Read the model definition and answer for the solid it produces. Units are mm, in the model's axes. A direction names the side the tool comes from. Coordinates: 2 decimals unless noted, no trailing zeros. Order: outer loops, then holes, each group sorted by start corner. A loop starts at its lowest first (then second) coordinate and runs counter-clockwise, first axis right, second up.
Autodesk Inventor part; units mm, degrees
ref_plane "작업 평면1" through (-21.25, -9.325, 0) normal (0, -1, 0) x (1, 0, 0)
ref_plane "YZ Plane" through (0, 0, 0) normal (1, 0, 0) x (0, 1, 0)
ref_plane "XZ Plane" through (0, 0, 0) normal (0, 1, 0) x (-1, 0, 0)
sketch "스케치1" plane through (0, 0, 0) normal (0, 0, 1) x (1, 0, 0)
  line L0 (-21.25, 18.125) -> (21.25, 18.125)
  line L1 (21.25, 18.125) -> (21.25, -18.125)
  line L2 (21.25, -18.125) -> (-21.25, -18.125)
  line L3 (-21.25, -18.125) -> (-21.25, 18.125)
  line L4 (-21.25, 18.125) -> (21.25, -18.125) construction
  line L5 (21.25, 18.125) -> (-21.25, -18.125) construction
  point P0 (0, 0)
  dimension "d0" = 42.5
  dimension "d1" = 36.25
extrude "돌출1" add sketch "스케치1" along normal blind 3
fillet "모깎기1" radius 5 2 edges at (21.25, 18.125, 1.5) (-21.25, 18.125, 1.5)
ref_plane "작업 평면1" through (-21.25, -9.325, 0) normal (0, -1, 0) x (1, 0, 0)
sketch "스케치2" plane through (-21.25, -9.325, 0) normal (0, -1, 0) x (1, 0, 0)
  line L0 (21.25, 0) -> (21.25, -4)
  circle A0 centre (21.25, -4) radius 2
  circle A1 centre (21.25, -4) radius 4
  line L1 (21.25, 0) -> (26.25, 0)
  line L2 (0, 0) -> (42.5, 0) construction
  line L3 (26.25, 0) -> (25.1524, -4.878)
  line L4 (21.25, 0) -> (16.25, 0)
  line L5 (16.25, 0) -> (17.4292, -5.184)
  dimension "d6" = 4
  dimension "d7" = 4
  dimension "d8" = 8
  dimension "d9" = 10
extrude "돌출2" add sketch "스케치2" along normal blind 2 contours L1 L3 A1 | A1 L5 | A1 L5 L4 picked at (20.9261, -0.7066)
pattern_linear "직사각형 패턴1" count 2 spacing 22.5 along (0, 1, 0) of "돌출2"
sketch "스케치3" plane through (0, 0, 0) normal (0, 0, -1) x (-1, 0, 0)
  circle A0 centre (16.825, -2.325) radius 4.425
  line L0 (21.25, -18.125) -> (-21.25, -18.125)
  line L1 (0, 0) -> (0, 4.3779)
  circle A1 centre (-16.825, -2.325) radius 4.425
  line L2 (21.25, 13.125) -> (21.25, -18.125)
  line L3 (-19.075, -0.075) -> (-14.575, -0.075)
  line L4 (-14.575, -0.075) -> (-14.575, -4.575)
  line L5 (-14.575, -4.575) -> (-19.075, -4.575)
  line L6 (-19.075, -4.575) -> (-19.075, -0.075)
  line L7 (-19.075, -0.075) -> (-14.575, -4.575) construction
  line L8 (-14.575, -0.075) -> (-19.075, -4.575) construction
  line L9 (14.575, -4.575) -> (19.075, -4.575)
  line L10 (19.075, -4.575) -> (19.075, -0.075)
  line L11 (19.075, -0.075) -> (14.575, -0.075)
  line L12 (14.575, -0.075) -> (14.575, -4.575)
  line L13 (14.575, -4.575) -> (19.075, -0.075) construction
  line L14 (19.075, -4.575) -> (14.575, -0.075) construction
  dimension "d16" = 15.8
  dimension "d17" = 33.65
  dimension "d18" = 4.5
  dimension "d19" = 4.5
  dimension "d20" = 4.5
  dimension "d21" = 4.5
extrude "돌출3" add sketch "스케치3" along normal blind 2
sketch "스케치4" plane through (0, 0, 3) normal (0, 0, 1) x (1, 0, 0)
  line L0 (-21.25, -18.125) -> (21.25, -18.125)
  line L1 (21.25, -18.125) -> (21.25, 13.125)
  line L2 (-21.25, 13.125) -> (-21.25, -18.125)
  line L3 (-21.25, -17.625) -> (21.25, -17.625)
  point P0 (0, 0)
  dimension "d24" = 0.5
extrude "돌출4" cut sketch "스케치4" against normal blind 3
sketch "스케치5" plane through (0, 0, 3) normal (0, 0, 1) x (1, 0, 0)
  line L0 (-17, 7) -> (-15, 7)
  line L1 (-15, 7) -> (-15, -13)
  line L2 (-15, -13) -> (-17, -13)
  line L3 (-17, -13) -> (-17, 7)
  line L4 (-17, 7) -> (-15, -13) construction
  line L5 (-15, 7) -> (-17, -13) construction
  point P0 (0, 0)
  point P1 (-16, -3)
  dimension "d27" = 2
  dimension "d28" = 20
  dimension "d32" = 3
  dimension "d37" = 16
extrude "돌출5" cut sketch "스케치5" against normal blind 0.5
chamfer "모따기1" distance 0.5 angle 45 4 edges at (-17, -3, 3) (-16, 7, 3) (-15, -3, 3) (-16, -13, 3)
sketch "스케치6" plane through (0, 0, 0) normal (0, 0, -1) x (-1, 0, 0)
  line L0 (14.575, -4.575) -> (19.075, -4.575)
  line L1 (19.075, -4.575) -> (19.075, -0.075)
  line L2 (19.075, -0.075) -> (14.575, -0.075)
  line L3 (14.575, -0.075) -> (14.575, -4.575)
  line L4 (-19.075, -0.075) -> (-19.075, -4.575)
  line L5 (-19.075, -4.575) -> (-14.575, -4.575)
  line L6 (-14.575, -4.575) -> (-14.575, -0.075)
  line L7 (-14.575, -0.075) -> (-19.075, -0.075)
  point P0 (0, 0)
extrude "돌출6" add sketch "스케치6" along normal blind 0.3
sketch "스케치7" plane through (-5, 11.175, 0) normal (0, -1, 0) x (1, 0, 0)
  arc A0 (1.1792, -5.184) -> (8.9024, -4.878) centre (5, -4) ccw
  line L0 (8.9024, -4.878) -> (1.1096, -4.878)
  line L1 (1.1096, -4.878) -> (1.1096, -8)
  line L2 (1.1096, -8) -> (8.9024, -8)
  line L3 (8.9024, -8) -> (8.9024, -4.878)
  line L4 (0, 0) -> (1.1792, -5.184)
  point P0 (5, 0)
  point P1 (5, -8)
extrude "돌출7" add sketch "스케치7" against normal blind 2 contours A0 L2 L1 L4 | A0 L3 L2
pattern_linear "직사각형 패턴2" count 2 spacing 22.5 along (0, -1, 0) of "돌출7"
chamfer "모따기2" distance 1 angle 45 4 edges at (3.9024, 12.175, -8) (-3.8904, 12.175, -8) (3.9024, -10.325, -8) (-3.8904, -10.325, -8)
properties part number "버튼 스위치 상단"
Q1. The part is cut by section D-D, the plane x = 15.5. Determine the outline of the cut face in (y, z) (3 decimals), then the cut area to 3 significant figures.
Q2. Determine the mould class of faces 5 (the flat face through (17, -2, -0.3)), 6 (the flat face through (-17, -5, -2)), 7 (the flat face through (-17, -0.075, -1)), 8 (the flat face through (3.4, 12.2, -7.5)) for opening direction X: +X half, -X half, draft (parallel to the pull), parting line (faces both ways), or undercut.
Q3. The part is cut by section A-A, the plane x = 0. Determine the outline of the cut face in (y, z) (3 decimals), then the cut area to 3 significant figures.
Q4. Each of these flat-tipped pins is pushed along its axis until it touches: P1, Ø1, axis at y = 11.5, z = -5.5, coming from the -X side; P2, Ø6.5, axis at x = 1, z = -4, coming from the -Y side (3 decimals); P3, Ø7, axis at x = 15, y = -2.5, coming from the -Z side; P4, Ø1.9, axis at y = -3, z = -1, coming from the +X side. Where does it stop, or does it pass through?
Q5. The part is cut by section B-B, the plane z = -3.5. Determine the outline of the cut face in (x, y) (1 decimal).
Q6. Which of the six approach directions +Z, -Z, +X, -X, +Y, -Y give full straight-line access (tool end or side, diameter ignored) to faces 1 (the flat face through (1, 13.175, -2)), 2 (the flat face through (1, -9.325, -2)), 3 (the flat face through (3.902, -10, -6)), 4 (the flat face through (-14.575, -2, -1))?
Q7. Straight lines are drawn through the part: L1, parallel to Z at x = 0, y = -10.5; L2, parallel to Y at x = -3, z = -5.75 (3 decimals); L3, parallel to Z at x = -17.5, y = -5.5. For each, find the intervals that lie inside material, in ascending order.
Computed values:
1. outline: (-17.625, 0) - (-6.547, 0) - (-6.547, -2) - (-4.575, -2) - (-4.575, -0.3) - (-0.075, -0.3) - (-0.075, -2) - (1.897, -2) - (1.897, 0) - (18.125, 0) - (18.125, 3) - (-17.625, 3) - close
1. area: 116 mm2
2. face 5: undercut
2. face 6: draft
2. face 7: undercut
2. face 8: +X half
3. outline: (-17.625, 0) - (-11.325, 0) - (-11.325, -2) - (-9.325, -2) - (-9.325, 0) - (11.175, 0) - (11.175, -2) - (13.175, -2) - (13.175, 0) - (18.125, 0) - (18.125, 3) - (-17.625, 3) - close; (-11.325, -8) - (-9.325, -8) - (-9.325, -6) - (-11.325, -6) - close; (11.175, -8) - (13.175, -8) - (13.175, -6) - (11.175, -6) - close
3. area: 123 mm2
4. P1: stops at x = -3.89
4. P2: stops at y = -11.325
4. P3: stops at z = -2
4. P4: stops at x = 21.25
5. outline: (-4.2, -11.3) - (-1.9, -11.3) - (-1.9, -9.3) - (-4.2, -9.3) - close; (-4.2, 11.2) - (-1.9, 11.2) - (-1.9, 13.2) - (-4.2, 13.2) - close; (1.9, -11.3) - (4.2, -11.3) - (4.2, -9.3) - (1.9, -9.3) - close; (1.9, 11.2) - (4.2, 11.2) - (4.2, 13.2) - (1.9, 13.2) - close
6. face 1: -Z, +X, -X, +Y
6. face 2: -Z, +X, -X
6. face 3: -Z, +X, +Y, -Y
6. face 4: -Z
7. L1: z = -8 to -6, -2 to 3
7. L2: y = -11.325 to -9.325, 11.175 to 13.175
7. L3: z = -2 to 3
